Source: CAD feature listing. Evaluate the final solid. Frame: model axes, mm. Face numbers are marked on the shaded views. A direction names the side the tool comes from. Give positions to 0.01 mm unless a question says otherwise; leave off trailing zeros. Order: outer loops, then holes, each group sorted by start corner. A loop starts at its lowest first (then second) coordinate and runs counter-clockwise, first axis right, second up. Notation, with made-up numbers: (-5.75, 44) -> (41.25, 44) arc R34 ccw to (41.25, 83) -> close; hole circle Ø10 at (31, -2.5). An arc over 180 degrees is marked (long way). Use CSV: the item, a comma, the result in double quotes.
Autodesk Inventor part; units mm, degrees
ref_plane "YZ Plane" through (0, 0, 0) normal (1, 0, 0) x (0, 1, 0)
ref_plane "XZ Plane" through (0, 0, 0) normal (0, 1, 0) x (-1, 0, 0)
ref_plane "XY Plane" through (0, 0, 0) normal (0, 0, 1) x (1, 0, 0)
sketch "Sketch1" plane through (0, 0, 0) normal (0, 1, 0) x (-1, 0, 0)
  line L0 (0, 0) -> (76.2, 152.4)
  line L1 (76.2, 152.4) -> (0, 152.4)
  line L2 (0, 152.4) -> (0, 0)
  dimension "d0" = 76.2
  dimension "d1" = 152.4
extrude "Extrusion1" add sketch "Sketch1" along normal blind 1.5875
sketch "Sketch2" plane through (0, 0, 0) normal (0, -1, 0) x (1, 0, 0)
  line L0 (-76.2, 152.4) -> (0, 152.4)
  line L1 (-74.4251, 152.4) -> (-3.175, 9.8998)
  line L2 (-3.175, 9.8998) -> (-4.5949, 9.1898)
  line L3 (0, 0) -> (-76.2, 152.4)
  line L4 (0, 0) -> (-76.2, 152.4)
  line L5 (0, 152.4) -> (0, 0)
  dimension "d4" = 1.5875
  dimension "d5" = 3.175
extrude "Extrusion2" add sketch "Sketch2" along normal blind 76.2 contours L0 L1 L2 L3
chamfer "Chamfer1" distance 14.2875 angle 45 1 edges at (0, 0.7937, 0)
chamfer "Chamfer2" distance 57.15 angle 63 1 edges at (-5.5958, -76.2, 12.9665)
sketch "Sketch4" plane through (-76.2, 1.5875, 152.4) normal (0, 0, 1) x (1, 0, 0)
  line L0 (0, 0) -> (1.5875, 0)
  line L1 (0, -77.7875) -> (18.2708, -77.7875)
  line L2 (0, -77.7875) -> (1.5875, -77.7875)
  line L3 (1.5875, -77.7875) -> (1.5875, -52.3875)
  line L4 (1.5875, -52.3875) -> (0, -52.3875)
  line L5 (0, -52.3875) -> (0, -77.7875)
  point P0 (76.2, -1.5875)
  dimension "d22" = 1.5875
  dimension "d23" = 25.4
extrude "Extrusion4" add sketch "Sketch4" along normal blind 25.4
sketch "Sketch5" plane through (-74.6125, -76.2, 152.4) normal (1, 0, 0) x (0, 0, -1)
  line L0 (0, 0) -> (-25.4, 0)
  line L1 (-25.4, 25.4) -> (-25.4, 0)
  point P0 (152.4, 76.2)
  point P1 (-19.05, 6.35)
  dimension "d24" = 6.35
  dimension "d25" = 6.35
hole "Hole1" at (-74.6125, -69.85, 171.45) direction (-1, 0, 0) diameter 5.1594 end through all
sketch "Sketch6" plane through (-6.3896, -19.05, 12.7791) normal (-0.8944272, 0, -0.4472136) x (-0.4472136, 0, 0.8944272)
  circle A0 centre (6.35, 14.2875) radius 3.175
  line L0 (0, 20.6375) -> (156.1009, 20.6375)
  line L1 (0, 0) -> (0, 20.6375)
  point P0 (-14.2875, 19.05)
  dimension "d33" = 6.35
  dimension "d34" = 6.35
  dimension "d35" = 6.35
extrude "Extrusion5" cut sketch "Sketch6" against normal blind 25.4
properties part number "15102898-16-P-0312"
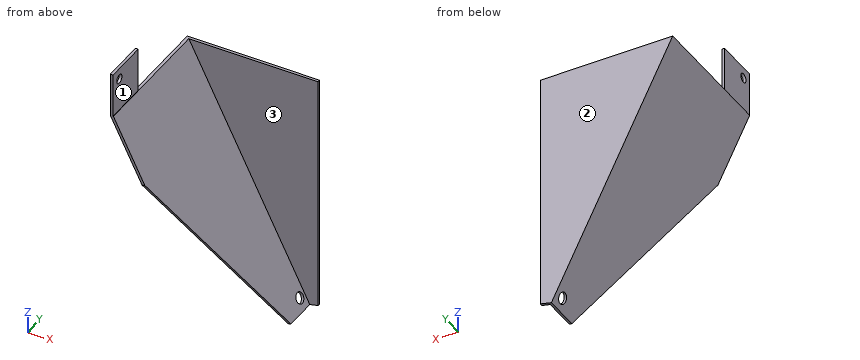
1. Section query B-B on y = -69.85. Return loops of the section in (x, z), plus the area to 3 significant figures.
Answer below:
outline,"(-76.2, 152.4) -> (-52.2, 104.41) -> (-50.62, 104.78) -> (-74.43, 152.4) -> (-74.61, 152.4) -> (-74.61, 168.87) -> (-76.2, 168.87) -> close; (-76.2, 174.03) -> (-74.61, 174.03) -> (-74.61, 177.8) -> (-76.2, 177.8) -> close"
area,"117 mm²"
2. Section query C-C on x = -53. Return loops of the section in (y, z), plus the area to 3 significant figures.
Answer below:
outline,"(-72.49, 109.55) -> (-70.73, 106) -> (1.59, 106) -> (1.59, 152.4) -> (0, 152.4) -> (0, 109.55) -> close"
area,"328 mm²"
3. Ray query, line 1 along Y through (x, z) = (-75.35, 171.45); line 2 along Y through (x, z) = (-55.5, 142); line 3 along Z through (x, y) = (-75.9, -69.85). Return the intervals inside material, ascending.
Answer below:
line 1,"y = -76.2 to -72.43, -67.27 to -50.8"
line 2,"y = 0 to 1.59"
line 3,"z = 151.8 to 168.87, 174.03 to 177.8"
4. Section query D-D on y = -11. Return loops of the section in (x, z).
Answer below:
outline,"(-76.2, 152.4) -> (-6.39, 12.78) -> (-4.8, 13.15) -> (-74.43, 152.4) -> close"
5. Pin query (flat end, axial travel): P1, Ø20.5, axis at y = -66, z = 165, coming from the +X side; P2, Ø1.7, axis at x = -75.5, z = 166.5, coming from the +Y side; P3, Ø1.5, axis at y = -21.5, z = 116, coming from the +X side. Return the tip coordinate at first contact, or that it passes through.
Answer below:
P1,"stops at x = -74.61"
P2,"stops at y = -50.8"
P3,"stops at x = -55.85"
6. Section query A-A on z = 171.45. Return loops of the section in (x, y).
Answer below:
outline,"(-76.2, -76.2) -> (-74.61, -76.2) -> (-74.61, -72.43) -> (-76.2, -72.43) -> close; (-76.2, -67.27) -> (-74.61, -67.27) -> (-74.61, -50.8) -> (-76.2, -50.8) -> close"
7. Access query for the marked faces 1, 2 and 3. Directions: +Z, -Z, +X, -X, +Y, -Y. A direction counts if a zero-diameter tool reaches every point of the face in a straight line with its end or side. Return the directions, or none.
Answer below:
face 1,"+Z, +X, +Y, -Y"
face 2,"+Z, -Z, +X, -X, +Y"
face 3,"+Z, +X, -Y"
